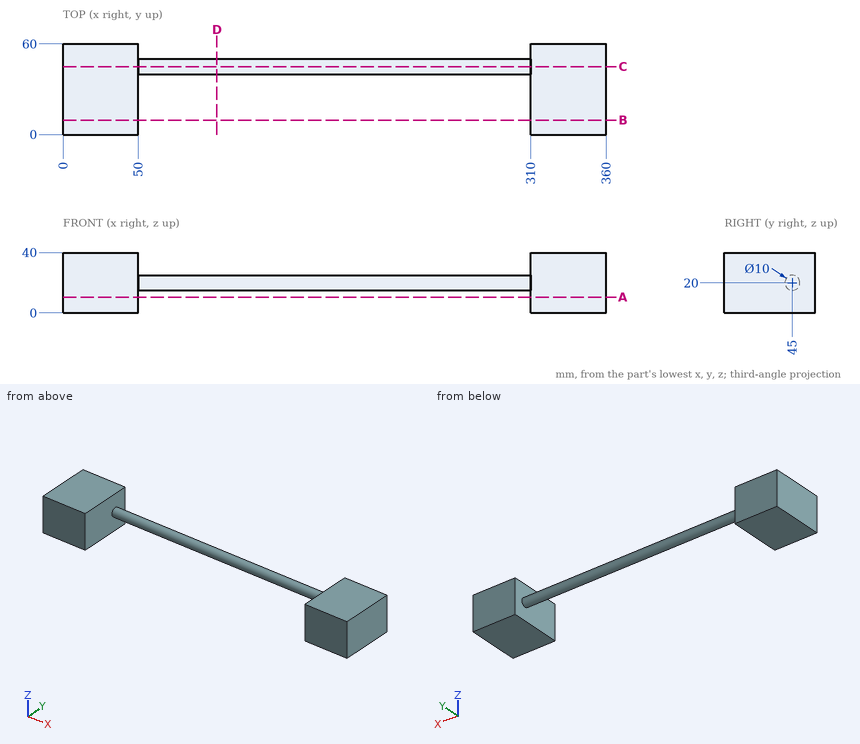
Could you check a few things on this drawing? It's one solid part, dimensions in mm from its lowest x, y, z. Round coordinates to 2 decimals unless told otherwise and drop trailing zeros. Order: outer loops, then holes, each group sorted by start corner. A loop starts at its lowest first (then second) coordinate and runs counter-clockwise, first axis right, second up.
(1) Imagine slicing it at D-D (x = 102). Write out the boundary of the cut face in (y, z), plus the area to 3 significant figures.
Response values:
outline: circle Ø10 at (45, 20)
area: 78.5 mm2
(2) Imagine slicing it at B-B (y = 9.5). Write out the boundary of the cut face in (x, z), plus the area to 3 significant figures.
Response values:
outline: (0, 0) - (50, 0) - (50, 40) - (0, 40) - close; (310, 0) - (360, 0) - (360, 40) - (310, 40) - close
area: 4,000 mm2
(3) Imagine slicing it at A-A (z = 10.5). Write out the boundary of the cut face in (x, y).
Response values:
outline: (0, 0) - (50, 0) - (50, 60) - (0, 60) - close; (310, 0) - (360, 0) - (360, 60) - (310, 60) - close
(4) Imagine slicing it at C-C (y = 45). Write out the boundary of the cut face in (x, z), plus the area to 3 significant figures.
Response values:
outline: (0, 0) - (50, 0) - (50, 15) - (310, 15) - (310, 0) - (360, 0) - (360, 40) - (310, 40) - (310, 25) - (50, 25) - (50, 40) - (0, 40) - close
area: 6,600 mm2
(5) Please list where these lines run through material, in increasing order: line 1 along X through (y, z) = (35.5, 13); line 2 along Y through (x, z) = (205, 18); line 3 along Y through (x, z) = (69.5, 21).
Response values:
line 1: x = 0 to 50, 310 to 360
line 2: y = 40.42 to 49.58
line 3: y = 40.1 to 49.9
(6) I'm going to push a flat-ended pin straight in: pin 1 (6 mm diameter, centred on x = 232, z = 25, fed in from -Y). Where does the tip first touch, or does it pass through?
Response values:
pin 1: stops at y = 40.42
